Check sheet for the modelled part. Datum: model origin and axes. Units: mm. Face numbers are marked on the shaded views. A direction names the side the tool comes from. Round coordinates to 2 decimals unless told otherwise and drop trailing zeros. Loops run counter-clockwise (first coordinate to the right, second up) from the corner with the lowest first, then second, coordinate; pieces in that order, holes last. Notation, with made-up numbers: (80.5, -36.75) - (127.5, -36.75) arc R11 cw to (127.5, -28.75) - close; hole circle Ø1 at (32, 25.5). An arc over 180 degrees is marked (long way). Return JSON: item names as keys, results as strings.
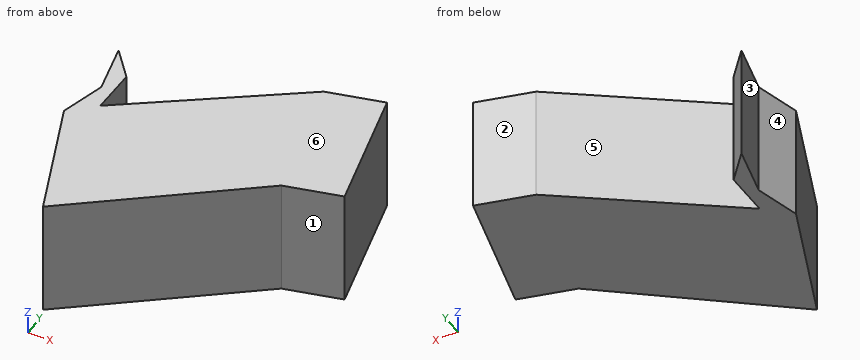
from build123d import *

# Parameters (mm, degrees)
F1_DEPTH = 25.4
F2_DEPTH = 25.4
F3_DEPTH = 25.4


with BuildPart() as f1:
    # F0 (on Top) → F1 (new body)
    with BuildSketch(Plane.XY):
        Polygon((5.3568482399, 62.3435284942), (0, 42.381696403), (22.1037119627, -13.7682110071), (96.1266011, 42.7341908216), (81.8468928337, 101.8667668104), (10.7136964798, 52.0066134632), (10.7136964798, 72.6804435253), (0, 85.6353342533), align=None)
    extrude(amount=F1_DEPTH)

    # F2 (add): a face of the model
    f2_faces = [f1.faces().sort_by_distance(p)[0] for p in [
        (47.6996824871, 44.5902490016, 25.4),
    ]]
    extrude(f2_faces, amount=F2_DEPTH)

    # F3 (add): a face of the model
    f3_faces = [f1.faces().sort_by_distance(p)[0] for p in [
        (88.9867469668, 72.300478816, 25.4),
    ]]
    extrude(f3_faces, amount=F3_DEPTH)


solid = f1.part
Q1. Scan lines: probe 1 along X at (y, z) = (67, 30); probe 2 along X at (y, z) = (80.5, 33.5); probe 3 along Y at (x, z) = (50, 26.5). Record each from-to range of solid material in increasing order. Write a range as [from, to].
Answer key:
{"probe 1": "x = [4.29, 10.71], [32.1, 116.4]", "probe 2": "x = [1.18, 4.25], [51.36, 113.14]", "probe 3": "y = [7.53, 79.54]"}
Q2. Draft check along Y on the marked faces 1, 2, 3 and 4. Enter one of: released by +Y, released by -Y, zero draft, split by the parting line, or undercut.
Answer key:
{"face 1": "released by -Y", "face 2": "released by +Y", "face 3": "undercut", "face 4": "undercut"}
Q3. Sectioned sample at D-D (y = 31). Enter the section's corners in (x, z).
Answer key:
{"outline": "(4.48, 0) - (80.75, 0) - (80.75, 50.8) - (4.48, 50.8) - close"}
Q4. Tool access check on the marked faces 5 and 6. Record the directions out of +Z, -Z, +X, -X, +Y, -Y that give a thin tool (end or side, any length) a straight path to the whole face; none if there is none.
Answer key:
{"face 5": "+Z, -Z, +Y", "face 6": "+Z, +X, -X, +Y, -Y"}
Q5. Sectioned sample at C-C (x = 13). Enter the section's corners in (y, z), plus the area to 3 significant figures.
Answer key:
{"outline": "(9.36, 0) - (53.61, 0) - (53.61, 50.8) - (9.36, 50.8) - close", "area": "2,250 mm²"}
Q6. Depth check by flat-ended pin: P1, Ø3, axis at y = 26.5, z = 6, coming from the +X side; P2, Ø6, axis at y = 57, z = 36.5, coming from the +X side; P3, Ø1, axis at y = 0.5, z = 35.5, coming from the -X side. Enter the tip coordinate at first touch or a pass-through.
Answer key:
{"P1": "stops at x = 76.82", "P2": "stops at x = 119.54", "P3": "stops at x = 16.29"}
Q7. Sectioned sample at A-A (y = 60). Enter the section's corners in (x, z).
Answer key:
{"outline": "(4.73, 0) - (10.71, 0) - (10.71, 50.8) - (4.73, 50.8) - close; (22.12, 0) - (118.09, 0) - (118.09, 50.8) - (22.12, 50.8) - close"}
Q8. Sectioned sample at B-B (z = 11.5). Enter the section's corners in (x, y), plus the area to 3 significant figures.
Answer key:
{"outline": "(0, 42.38) - (22.1, -13.77) - (96.13, 42.73) - (120.82, 48.7) - (106.54, 107.83) - (81.85, 101.87) - (10.71, 52.01) - (10.71, 72.68) - (0, 85.64) - (5.36, 62.34) - close", "area": "7,390 mm²"}
